from build123d import *

# Parameters (mm, degrees)
BOSS_EXTRUDE1_DEPTH = 6.35
SKETCH2_W           = 25.4
SKETCH2_H           = 6.35
CUT_EXTRUDE1_DEPTH  = 6.35
SKETCH3_W           = 25.4
SKETCH3_H           = 6.35
CUT_EXTRUDE2_DEPTH  = 6.35
SKETCH4_R           = 1.5875
CUT_EXTRUDE4_DEPTH  = 6.35


with BuildPart() as part:
    # Sketch1 → Boss-Extrude1 (new body)
    with BuildSketch(Plane.XY):
        Polygon((6.35, 38.1), (0, 38.1), (0, 25.4), (0, 12.7), (0, 0), (6.35, 0), (146.05, 0), (152.4, 0), (152.4, 12.7), (152.4, 25.4), (152.4, 38.1), (146.05, 38.1), align=None)
    extrude(amount=BOSS_EXTRUDE1_DEPTH)

    # Sketch2 → Cut-Extrude1 (cut)
    with BuildSketch(Plane.XY.offset(6.35)):
        with Locations((25.4, 12.7)):
            Rectangle(SKETCH2_W, SKETCH2_H)
    extrude(amount=-CUT_EXTRUDE1_DEPTH, mode=Mode.SUBTRACT)

    # Sketch3 → Cut-Extrude2 (cut)
    with BuildSketch(Plane.XY.offset(6.35)):
        with Locations((127, 12.7)):
            Rectangle(SKETCH3_W, SKETCH3_H)
    extrude(amount=-CUT_EXTRUDE2_DEPTH, mode=Mode.SUBTRACT)

    # Sketch4 → Cut-Extrude4 (cut)
    with BuildSketch(Plane.XY.offset(6.35)):
        with Locations((76.2, 28.575)):
            Circle(SKETCH4_R)
    extrude(amount=-CUT_EXTRUDE4_DEPTH, mode=Mode.SUBTRACT)


solid = part.part
The listing builds one solid part. Answer for the finished solid, in the listing's coordinates (mm). A direction names the side the tool comes from. Give positions to 0.01 mm unless a question says otherwise; leave off trailing zeros. Write each loop counter-clockwise with the first axis right and the second up, starting at its lowest first coordinate (ties: lowest second). Pieces come first, ordered by that corner, then holes. Notation, with made-up numbers: (70.25, 36.5) - (103.25, 36.5) arc R15 cw to (103.25, 46.5) - close; hole circle Ø9 at (29, 7.25). An arc over 180 degrees is marked (long way). One line per question, with ' | ' between items. Start each with the question number.
1. Section C-C, the plane z = 3.25 is taken. Determine the outline of the cut face in (x, y) (1 decimal), then the cut area to 3 significant figures.
2. For faces 1 (the face through (0, 19, 3)), 2 (the face through (139.7, 13, 3)), determine the directions among +Z, -Z, +X, -X, +Y, -Y from which every point of the face is accessible in a straight line to the end or side of a thin tool.
3. Straight lines are drawn through the part: line 1 (X direction, y = 14.5, z = 5.5); line 2 (Y direction, x = 16, z = 2.75) (3 decimals); line 3 (X direction, y = 29.5, z = 4.5). For each, find the intervals that lie inside material, in ascending order.
4. Section D-D, the plane x = 15.5 is taken. Determine the outline of the cut face in (y, z) (3 decimals).
5. Section A-A, the plane x = 76.2 is taken. Determine the outline of the cut face in (y, z), then the cut area to 3 significant figures.
6. Section B-B, the plane y = 13.5 is taken. Determine the outline of the cut face in (x, z).
7. Determine the mould class of faces 3 (the face through (77, 38.1, 3)), 4 (the face through (25, 15.875, 3)), 5 (the face through (75, 19, 6.35)) for opening direction Y: +Y half, -Y half, draft (parallel to the pull), parting line (faces both ways), or undercut.
Result:
1) outline: (0, 0) - (152.4, 0) - (152.4, 38.1) - (0, 38.1) - close; hole (12.7, 9.5) - (38.1, 9.5) - (38.1, 15.9) - (12.7, 15.9) - close; hole circle Ø3.2 at (76.2, 28.6); hole (114.3, 9.5) - (139.7, 9.5) - (139.7, 15.9) - (114.3, 15.9) - close | area: 5,480 mm2
2) face 1: +Z, -Z, -X, +Y, -Y | face 2: +Z, -Z
3) line 1: x = 0 to 12.7, 38.1 to 114.3, 139.7 to 152.4 | line 2: y = 0 to 9.525, 15.875 to 38.1 | line 3: x = 0 to 74.91, 77.49 to 152.4
4) outline: (0, 0) - (9.525, 0) - (9.525, 6.35) - (0, 6.35) - close; (15.875, 0) - (38.1, 0) - (38.1, 6.35) - (15.875, 6.35) - close
5) outline: (0, 0) - (26.99, 0) - (26.99, 6.35) - (0, 6.35) - close; (30.16, 0) - (38.1, 0) - (38.1, 6.35) - (30.16, 6.35) - close | area: 222 mm2
6) outline: (0, 0) - (12.7, 0) - (12.7, 6.35) - (0, 6.35) - close; (38.1, 0) - (114.3, 0) - (114.3, 6.35) - (38.1, 6.35) - close; (139.7, 0) - (152.4, 0) - (152.4, 6.35) - (139.7, 6.35) - close
7) face 3: +Y half | face 4: undercut | face 5: draft
